from build123d import *

# Parameters (mm, degrees)
SKETCH_1_W          = 108
SKETCH_1_H          = 138
EXTRUDE_1_DEPTH     = 4
SKETCH_3_W          = 108
SKETCH_3_H          = 138
CUT_EXTRUDE_2_DEPTH = 1
SKETCH_4_W          = 10
SKETCH_4_H          = 3
EXTRUDE_2_DEPTH     = 6
SKETCH_5_W          = 10
SKETCH_5_H          = 3
SKETCH_5_W_2        = 15
EXTRUDE_3_DEPTH     = 6
SKETCH_6_W          = 15
SKETCH_6_H          = 3
SKETCH_6_W_2        = 10
EXTRUDE_4_DEPTH     = 6
SKETCH_7_W          = 10
SKETCH_7_H          = 3
EXTRUDE_5_DEPTH     = 6
SKETCH_8_W          = 6
SKETCH_8_H          = 3
EXTRUDE_6_DEPTH     = 0.2
SKETCH_9_W          = 6
SKETCH_9_H          = 3
EXTRUDE_7_DEPTH     = 0.2
SKETCH_10_W         = 6
SKETCH_10_H         = 3
EXTRUDE_8_DEPTH     = 0.2
SKETCH_11_W         = 6
SKETCH_11_H         = 3
EXTRUDE_9_DEPTH     = 0.2
SKETCH_12_W         = 6
SKETCH_12_H         = 3
EXTRUDE_10_DEPTH    = 0.2


with BuildPart() as part:
    # Эскиз1 → Бобышка-Вытянуть1 (new body)
    with BuildSketch(Plane(origin=(0, 0, 0), x_dir=(1, 0, 0), z_dir=(0, 1, 0))):
        with Locations((54, -69)):
            Rectangle(SKETCH_1_W, SKETCH_1_H)
    extrude(amount=EXTRUDE_1_DEPTH)

    # Эскиз3 → Вырез-Вытянуть2 (cut)
    with BuildSketch(Plane.XZ):
        with Locations((54, 69)):
            Rectangle(SKETCH_3_W, SKETCH_3_H)
    extrude(amount=-CUT_EXTRUDE_2_DEPTH, mode=Mode.SUBTRACT)

    # Эскиз4 → Бобышка-Вытянуть2 (add)
    with BuildSketch(Plane.XY.offset(138)):
        with Locations((15, 2.5)):
            Rectangle(SKETCH_4_W, SKETCH_4_H)
        with Locations((35, 2.5)):
            Rectangle(SKETCH_4_W, SKETCH_4_H)
        with Locations((55, 2.5)):
            Rectangle(SKETCH_4_W, SKETCH_4_H)
        with Locations((75, 2.5)):
            Rectangle(SKETCH_4_W, SKETCH_4_H)
        with Locations((95, 2.5)):
            Rectangle(SKETCH_4_W, SKETCH_4_H)
    extrude(amount=EXTRUDE_2_DEPTH)

    # Эскиз5 → Бобышка-Вытянуть3 (add)
    with BuildSketch(Plane.ZY):
        with Locations((14, 2.5)):
            Rectangle(SKETCH_5_W, SKETCH_5_H)
        with Locations((126.5, 2.5)):
            Rectangle(SKETCH_5_W_2, SKETCH_5_H)
    extrude(amount=EXTRUDE_3_DEPTH)

    # Эскиз6 → Бобышка-Вытянуть4 (add)
    with BuildSketch(Plane(origin=(108, 0, 0), x_dir=(0, 0, -1), z_dir=(1, 0, 0))):
        with Locations((-126.5, 2.5)):
            Rectangle(SKETCH_6_W, SKETCH_6_H)
        with Locations((-14, 2.5)):
            Rectangle(SKETCH_6_W_2, SKETCH_6_H)
    extrude(amount=EXTRUDE_4_DEPTH)

    # Эскиз7 → Бобышка-Вытянуть5 (add)
    with BuildSketch(Plane(origin=(0, 0, 0), x_dir=(-1, 0, 0), z_dir=(0, 0, -1))):
        with Locations((-94, 2.5)):
            Rectangle(SKETCH_7_W, SKETCH_7_H)
        with Locations((-74, 2.5)):
            Rectangle(SKETCH_7_W, SKETCH_7_H)
        with Locations((-54, 2.5)):
            Rectangle(SKETCH_7_W, SKETCH_7_H)
        with Locations((-34, 2.5)):
            Rectangle(SKETCH_7_W, SKETCH_7_H)
        with Locations((-14, 2.5)):
            Rectangle(SKETCH_7_W, SKETCH_7_H)
    extrude(amount=EXTRUDE_5_DEPTH)

    # Эскиз8 → Бобышка-Вытянуть6 (add)
    with BuildSketch(Plane.ZY.offset(-10)):
        with Locations((141, 2.5)):
            Rectangle(SKETCH_8_W, SKETCH_8_H)
    extrude(amount=EXTRUDE_6_DEPTH)

    # Эскиз9 → Бобышка-Вытянуть7 (add)
    with BuildSketch(Plane.ZY.offset(-30)):
        with Locations((141, 2.5)):
            Rectangle(SKETCH_9_W, SKETCH_9_H)
    extrude(amount=EXTRUDE_7_DEPTH)

    # Эскиз10 → Бобышка-Вытянуть8 (add)
    with BuildSketch(Plane.ZY.offset(-50)):
        with Locations((141, 2.5)):
            Rectangle(SKETCH_10_W, SKETCH_10_H)
    extrude(amount=EXTRUDE_8_DEPTH)

    # Эскиз11 → Бобышка-Вытянуть9 (add)
    with BuildSketch(Plane.ZY.offset(-70)):
        with Locations((141, 2.5)):
            Rectangle(SKETCH_11_W, SKETCH_11_H)
    extrude(amount=EXTRUDE_9_DEPTH)

    # Эскиз12 → Бобышка-Вытянуть10 (add)
    with BuildSketch(Plane.ZY.offset(-90)):
        with Locations((141, 2.5)):
            Rectangle(SKETCH_12_W, SKETCH_12_H)
    extrude(amount=EXTRUDE_10_DEPTH)


solid = part.part
Input: part model. Units: mm. Frame: model coordinates. A direction names the side the tool comes from. Coordinates: 2 decimals unless noted, no trailing zeros. Order: outer loops, then holes, each group sorted by start corner. A loop starts at its lowest first (then second) coordinate and runs counter-clockwise, first axis right, second up. Notation, with made-up numbers: M -5.5,56 L 42.5,56 A27 ccw 42.5,84 Z; hole C 41.5,41.25 d10. An arc over 180 degrees is marked long. One line per question, with ' | ' between items.
Item 1: Section B-B (z = 55.5). Output: boundary loops of the cut face in (x, y).
Geometry results:
outline: M 0,1 L 108,1 L 108,4 L 0,4 Z
Item 2: Section A-A (x = 26.5). Output: boundary loops of the cut face in (y, z), then the cut area to 3 significant figures.
Geometry results:
outline: M 1,0 L 4,0 L 4,138 L 1,138 Z | area: 414 mm^2
Item 3: Pin query (flat end, axial travel): pin 1 (0.9 mm diameter, centred on x = 85, y = 3, fed in from -Z); pin 2 (0.9 mm diameter, centred on y = 3, z = 45.5, fed in from -X); pin 3 (0.9 mm diameter, centred on y = 2.5, z = 140, fed in from +X). Return the tip coordinate at first contact, or that it passes through.
Geometry results:
pin 1: stops at z = 0 | pin 2: stops at x = 0 | pin 3: stops at x = 100
Item 4: Draft query along X for faces 1 (the flat face through (54, 3, -6)), 2 (the flat face through (79, 2, -3)), 3 (the flat face through (40, 2, 141)), 4 (the flat face through (114, 3, 14)). Return one class per face: released by +X, released by -X, zero draft, split by the parting line, or undercut.
Geometry results:
face 1: zero draft | face 2: undercut | face 3: undercut | face 4: released by +X
Item 5: Reachability of faces 5 (the flat face through (45, 2, 138)), 6 (the flat face through (59, 2, -3)), 7 (the flat face through (-3, 2, 9)) from +Z, -Z, +X, -X, +Y, -Y: full face, straight path, thin tool, end or side. Return the list, or none.
Geometry results:
face 5: +Z, +Y, -Y | face 6: -Z, +Y, -Y | face 7: -Z, -X, +Y, -Y
Item 6: Ray query, line 1 along Z through (x, y) = (63, 2.75); line 2 along X through (y, z) = (2.6, 39.5). Return the intervals inside material, ascending.
Geometry results:
line 1: z = 0 to 138 | line 2: x = 0 to 108
